Build history of the part. All positions in model axes, mm. Face numbers are marked on the shaded views. Round coordinates to 2 decimals unless told otherwise and drop trailing zeros. Write each question's results on one line, items separated by ' | '. Start each with the question number.
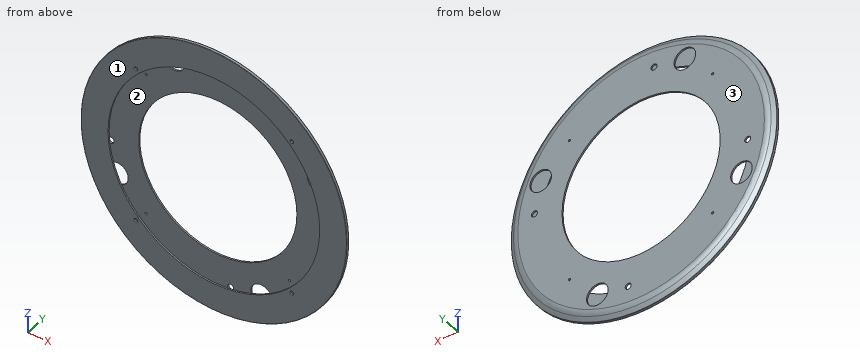
```python
from build123d import *

# Parameters (mm, degrees)
SKETCH_3_R          = 14.325286012
CUT_EXTRUDE_2_DEPTH = 3
SKETCH_4_R          = 4
CUT_EXTRUDE_3_DEPTH = 3
SKETCH_5_R          = 2.5
CUT_EXTRUDE_4_DEPTH = 2
SKETCH_6_R          = 1.5
CUT_EXTRUDE_5_DEPTH = 3


with BuildPart() as part:
    # 草图1 → 旋转1 (revolve)
    with BuildSketch(Plane.XY):
        with BuildLine():
            Line((163.684919254, 9), (105, 9))
            Line((105, 9), (105, 7))
            Line((105, 7), (163.684919254, 7))
            ThreePointArc((163.684919254, 7), (165.90837568, 6.859208887), (168.096314472, 6.439084553))
            Line((168.096314472, 6.439084553), (174.5, 2.656413608))
            Line((174.5, 2.656413608), (174.5, 2))
            Line((174.5, 2), (140.5, 2))
            Line((140.5, 2), (140.5, 0))
            Line((140.5, 0), (176, 0))
            ThreePointArc((176, 0), (176.353553391, 0.146446609), (176.5, 0.5))
            Line((176.5, 0.5), (176.5, 3.231140782))
            ThreePointArc((176.5, 3.231140782), (176.435661844, 3.476495133), (176.259204971, 3.658706898))
            Line((176.259204971, 3.658706898), (171.019179277, 6.835386852))
            ThreePointArc((171.019179277, 6.835386852), (167.508429427, 8.447549196), (163.684919254, 9))
        make_face()
    revolve(axis=Axis((0, 0, 0), (0, -1, 0)))

    # 草图3 → 切除-拉伸2 (cut)
    with BuildSketch(Plane(origin=(0, 9, 0), x_dir=(1, 0, 0), z_dir=(0, 1, 0))):
        with Locations((58.081681413, 133.219094668)):
            Circle(SKETCH_3_R)
        with Locations((133.219094668, -58.081681413)):
            Circle(SKETCH_3_R)
        with Locations((-58.081681413, -133.219094668)):
            Circle(SKETCH_3_R)
        with Locations((-133.219094668, 58.081681413)):
            Circle(SKETCH_3_R)
    extrude(amount=-CUT_EXTRUDE_2_DEPTH, mode=Mode.SUBTRACT)

    # 草图4 → 切除-拉伸3 (cut)
    with BuildSketch(Plane(origin=(0, 9, 0), x_dir=(1, 0, 0), z_dir=(0, 1, 0))):
        with Locations((17.053492548, 141.497897625)):
            Circle(SKETCH_4_R)
        with Locations((141.497897625, -17.053492548)):
            Circle(SKETCH_4_R)
        with Locations((-17.053492548, -141.497897625)):
            Circle(SKETCH_4_R)
        with Locations((-141.497897625, 17.053492548)):
            Circle(SKETCH_4_R)
    extrude(amount=-CUT_EXTRUDE_3_DEPTH, mode=Mode.SUBTRACT)

    # 草图5 → 切除-拉伸4 (cut)
    with BuildSketch(Plane.XZ):
        with Locations((-103.5, 103.5)):
            Circle(SKETCH_5_R)
        with Locations((103.5, 103.5)):
            Circle(SKETCH_5_R)
        with Locations((103.5, -103.5)):
            Circle(SKETCH_5_R)
        with Locations((-103.5, -103.5)):
            Circle(SKETCH_5_R)
    extrude(amount=-CUT_EXTRUDE_4_DEPTH, mode=Mode.SUBTRACT)

    # 草图6 → 切除-拉伸5 (cut)
    with BuildSketch(Plane(origin=(0, 9, 0), x_dir=(1, 0, 0), z_dir=(0, 1, 0))):
        with Locations((-95, 95)):
            Circle(SKETCH_6_R)
        with Locations((95, 95)):
            Circle(SKETCH_6_R)
        with Locations((95, -95)):
            Circle(SKETCH_6_R)
        with Locations((-95, -95)):
            Circle(SKETCH_6_R)
    extrude(amount=-CUT_EXTRUDE_5_DEPTH, mode=Mode.SUBTRACT)


solid = part.part
```
1. Wall check: line 1 (Y direction, x = 121.5, z = -73); line 2 (Z direction, x = 103.5, y = 0.7); line 3 (X direction, y = 2.75, z = -67). Give the ranges that are in metal, low to high. Write a range as from..to.
2. Flat gauge pins, fed straight in: pin 1 Ø5 at (x, z) = (17.05, -141.5) entering from +Y; pin 2 Ø3 at (x, y) = (107.5, 4.5) entering from -Z; pin 3 Ø6 at (x, z) = (-7.5, 113.5) entering from -Y. Where does each tip first touch, or does it go through?
3. Cut at A-A (x = 60). Give the number of separate pieces and of enclosed holes in the cut face, plus the area to 3 significant figures.
4. Mould opens along Y. For the marked faces 1, 2 and 3 say: pulls with the +Y half, pulls with the -Y half, needs draft (parallel to the pull), parting line crosses it, or undercut.
A:
1) line 1: y = 0..2, 7..9 | line 2: z = -142.97..-106, -101..-95.02, 95.02..101, 106..142.97 | line 3: x = -163.29..-160.95, 160.95..163.29
2) pin 1: stops at y = 2 | pin 2: stops at z = -140.74 | pin 3: stops at y = 7
3) separate pieces: 3 | enclosed holes: 0 | area: 419 mm^2
4) face 1: pulls with the -Y half | face 2: undercut | face 3: pulls with the +Y half
